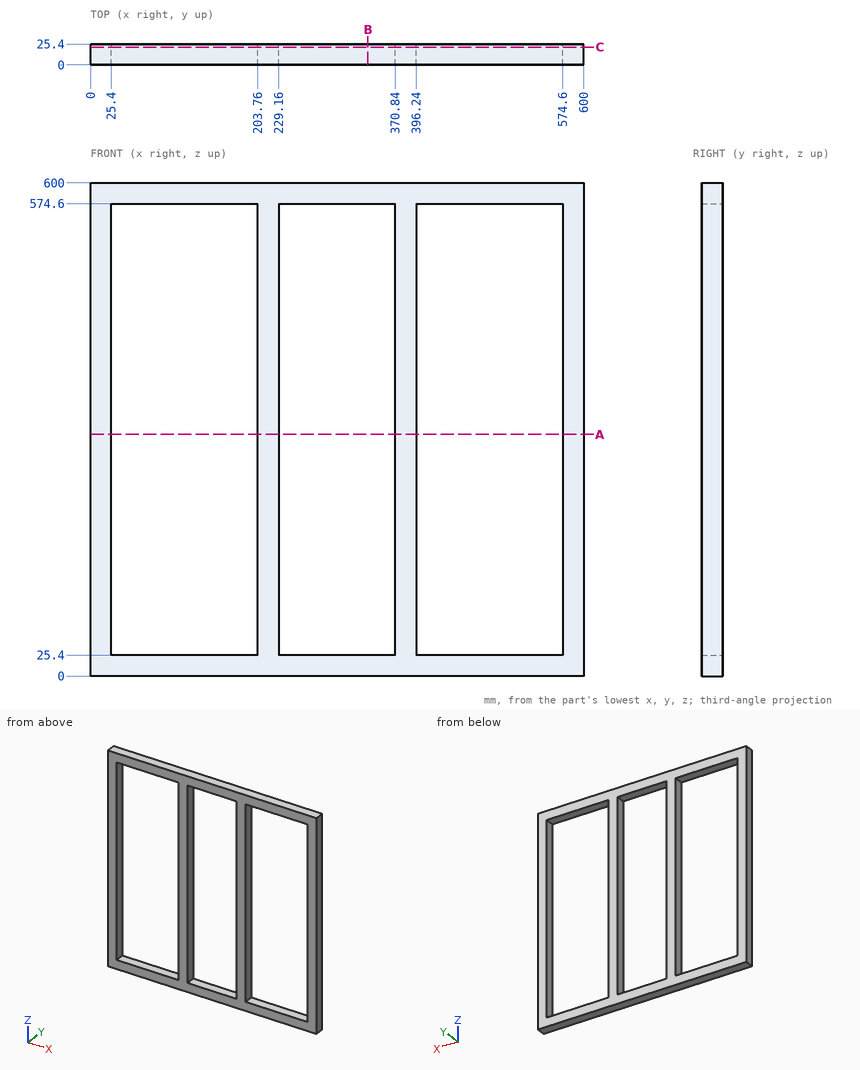
Geometry check sheet. Reference: drawing and pictorial views, mm from the part's lowest x, y, z. Coordinates: 2 decimals unless noted, no trailing zeros. Loops run counter-clockwise (first coordinate to the right, second up) from the corner with the lowest first, then second, coordinate; pieces in that order, holes last. Notation, with made-up numbers: (-6, 22) -> (13, 22) arc R20 ccw to (13, 44) -> close; hole circle Ø9 at (-19.75, 43). An arc over 180 degrees is marked (long way). Write item = value, one per line. Start each with the question number.
1. Section check C-C on y = 21.5. Record the cut outline in (x, z).
2. Section check B-B on x = 337.5. Record the cut outline in (y, z).
3. Section check A-A on z = 294. Record the cut outline in (x, y), then the cut area to 3 significant figures.
4. Depth check by flat-ended pin: P1, Ø1, axis at y = 19, z = 371, coming from the -X side; P2, Ø8, axis at x = 403, z = 302.5, coming from the -Y side. Enter the tip coordinate at first touch or a pass-through.
5. Material ranges on line 1 (X direction, y = 21.75, z = 193); line 2 (Z direction, x = 233.5, y = 16.75), recorded low to high.
Responses:
q1.outline = (0, 0) -> (600, 0) -> (600, 600) -> (0, 600) -> close; hole (25.4, 25.4) -> (203.76, 25.4) -> (203.76, 574.6) -> (25.4, 574.6) -> close; hole (229.16, 25.4) -> (370.84, 25.4) -> (370.84, 574.6) -> (229.16, 574.6) -> close; hole (396.24, 25.4) -> (574.6, 25.4) -> (574.6, 574.6) -> (396.24, 574.6) -> close
q2.outline = (0, 0) -> (25.4, 0) -> (25.4, 25.4) -> (0, 25.4) -> close; (0, 574.6) -> (25.4, 574.6) -> (25.4, 600) -> (0, 600) -> close
q3.outline = (0, 0) -> (25.4, 0) -> (25.4, 25.4) -> (0, 25.4) -> close; (203.76, 0) -> (229.16, 0) -> (229.16, 25.4) -> (203.76, 25.4) -> close; (370.84, 0) -> (396.24, 0) -> (396.24, 25.4) -> (370.84, 25.4) -> close; (574.6, 0) -> (600, 0) -> (600, 25.4) -> (574.6, 25.4) -> close
q3.area = 2,580 mm2
q4.P1 = 0
q4.P2 = through
q5.line_1 = 0 to 25.4, 203.76 to 229.16, 370.84 to 396.24, 574.6 to 600
q5.line_2 = 0 to 25.4, 574.6 to 600
